Autodesk Inventor part; units mm, degrees
ref_plane "YZ Plane" through (0, 0, 0) normal (1, 0, 0) x (0, 1, 0)
ref_plane "XZ Plane" through (0, 0, 0) normal (0, 1, 0) x (-1, 0, 0)
ref_plane "XY Plane" through (0, 0, 0) normal (0, 0, 1) x (1, 0, 0)
sketch "スケッチ1" plane through (0, 0, 0) normal (0, 0, 1) x (1, 0, 0)
  circle A0 centre (0, 0) radius 6
  dimension "d0" = 12
extrude "押し出し1" add sketch "スケッチ1" along normal blind 100
sketch "スケッチ2" plane through (0, 0, 0) normal (1, 0, 0) x (0, 1, 0)
  line L0 (0, 0) -> (0, 100)
  line L1 (6, 100) -> (-6, 100)
  point P0 (0, 75)
  point P1 (0, 25)
  point P2 (0, 50)
  dimension "d3" = 25
  dimension "d4" = 25
hole "穴1" at (0, 0, 75) at (0, 0, 25) direction (-1, 0, 0) diameter 3.2 end through all both
sketch "スケッチ3" plane through (0, 0, 0) normal (1, 0, 0) x (0, 1, 0)
  line L0 (0, 0) -> (0, 100)
  line L1 (6, 100) -> (-6, 100)
  line L2 (6, 0) -> (-6, 0)
  point P0 (0, 95)
  point P1 (0, 5)
  dimension "d12" = 5
  dimension "d13" = 5
hole "穴2" at (0, 0, 95) at (0, 0, 5) direction (-1, 0, 0) diameter 2.2 end through all both
properties part number "xx_jiku_kakudo"
Could you check a few things on this model? Use its own coordinates, in mm. Coordinates: 2 decimals unless noted, no trailing zeros. Order: outer loops, then holes, each group sorted by start corner. A loop starts at its lowest first (then second) coordinate and runs counter-clockwise, first axis right, second up. Notation, with made-up numbers: (23.5, -36) -> (53.5, -36) arc R8 ccw to (53.5, -27) -> close; hole circle Ø8 at (-24, 85.25). An arc over 180 degrees is marked (long way). One line per question, with ' | ' between items.
Q1. I'm going to push flat-ended pins straight in: P1, Ø6, axis at y = 4.5, z = 34, coming from the +X side; P2, Ø4, axis at x = -4, z = 23, coming from the +Y side; P3, Ø1, axis at y = 4, z = 79.5, coming from the +X side. Where does each tip first touch, or does it pass through?
Return value:
P1: x = 5.81 | P2: y = 5.66 | P3: x = 4.87
Q2. If I drill on L1, parallel to Z at x = -2.75, y = 0; L2, parallel to Z at x = 3, y = 0.5; L3, parallel to Z at x = -3.25, y = 1.25, over which ranges is the centre line in solid material (lowest first)?
Return value:
L1: 0 to 3.9, 6.1 to 23.4, 26.6 to 73.4, 76.6 to 93.9, 96.1 to 100 | L2: 0 to 4.02, 5.98 to 23.48, 26.52 to 73.48, 76.52 to 94.02, 95.98 to 100 | L3: 0 to 24, 26 to 74, 76 to 100
Q3. Imagine slicing it at C-C on z = 95. Please give me the cut outline in (x, y), and give its area (3 significant figures).
Return value:
outline: (-5.9, -1.1) arc R6 ccw to (5.9, -1.1) -> close; (-5.9, 1.1) -> (5.9, 1.1) arc R6 ccw to start | area: 86.8 mm²
Q4. Imagine slicing it at D-D on z = 82. Please give me the cut outline in (x, y), and give its area (3 significant figures).
Return value:
outline: circle Ø12 at (0, 0) | area: 113 mm²
Q5. Thinking about a two-plate mould opening in Y: for faces 1 (the face through (5.723, -1.802, 49.3)), 2 (the face through (0, 0, 0)), 3 (the face through (-0.08, -1.08, 26.18)), which applies, pulls with the +Y half, pulls with the -Y half, needs draft (parallel to the pull), parting line crosses it, or undercut?
Return value:
face 1: parting line crosses it | face 2: needs draft | face 3: undercut
Q6. Imagine slicing it at B-B on x = -2.25. Please give me the cut outline in (y, z), and give its area (3 significant figures).
Return value:
outline: (-5.56, 0) -> (5.56, 0) -> (5.56, 100) -> (-5.56, 100) -> close; hole circle Ø3.2 at (0, 25); hole circle Ø3.2 at (0, 75); hole circle Ø2.2 at (0, 5); hole circle Ø2.2 at (0, 95) | area: 1,090 mm²
Q7. Imagine slicing it at A-A on y = 0. Please give me the cut outline in (x, z), and give its area (3 significant figures).
Return value:
outline: (-6, 0) -> (6, 0) -> (6, 3.9) -> (-6, 3.9) -> close; (-6, 6.1) -> (6, 6.1) -> (6, 23.4) -> (-6, 23.4) -> close; (-6, 26.6) -> (6, 26.6) -> (6, 73.4) -> (-6, 73.4) -> close; (-6, 76.6) -> (6, 76.6) -> (6, 93.9) -> (-6, 93.9) -> close; (-6, 96.1) -> (6, 96.1) -> (6, 100) -> (-6, 100) -> close | area: 1,070 mm²
